Geometry: final body of the model. Coordinates: model frame, mm. A direction names the side the tool comes from. Round coordinates to 2 decimals unless told otherwise and drop trailing zeros. Write each loop counter-clockwise with the first axis right and the second up, starting at its lowest first coordinate (ties: lowest second). Pieces come first, ordered by that corner, then holes. Notation, with made-up numbers: (10.5, 1.25) - (30.5, 1.25) arc R22 cw to (30.5, 25.25) - close; hole circle Ø3 at (85.25, -38). An arc over 180 degrees is marked (long way). Use a Markdown table: item, result. Add a question column.
```python
from build123d import *

# Parameters (mm, degrees)
F0_W     = 3.175
F0_H     = 3.175
F0_H_2   = 6.35
F0_W_2   = 12.7
F1_DEPTH = 3.175
F2_W     = 19.05
F2_H     = 3.175
F3_DEPTH = 6.35
F4_W     = 6.35
F4_H     = 3.175
F5_DEPTH = 25.4


with BuildPart() as f1:
    # F0 (on Top) → F1 (new body)
    with BuildSketch(Plane.XY):
        with Locations((1.5875, 1.5875)):
            Rectangle(F0_W, F0_H)
        with Locations((1.5875, 6.35)):
            Rectangle(F0_W, F0_H_2)
        with Locations((1.5875, 11.1125)):
            Rectangle(F0_W, F0_H)
        with Locations((1.5875, 15.875)):
            Rectangle(F0_W, F0_H_2)
        with Locations((9.525, 11.1125)):
            Rectangle(F0_W_2, F0_H)
        with Locations((1.5875, 20.6375)):
            Rectangle(F0_W, F0_H)
        with Locations((17.4625, 6.35)):
            Rectangle(F0_W, F0_H_2)
        with Locations((17.4625, 11.1125)):
            Rectangle(F0_W, F0_H)
        with Locations((1.5875, 23.8125)):
            Rectangle(F0_W, F0_H)
        with Locations((9.525, 20.6375)):
            Rectangle(F0_W_2, F0_H)
        with Locations((17.4625, 15.875)):
            Rectangle(F0_W, F0_H_2)
        with Locations((17.4625, 1.5875)):
            Rectangle(F0_W, F0_H)
        with Locations((17.4625, 20.6375)):
            Rectangle(F0_W, F0_H)
        with Locations((17.4625, 23.8125)):
            Rectangle(F0_W, F0_H)
    extrude(amount=F1_DEPTH)

    # F2 (on face) → F3 (join)
    with BuildSketch(Plane(origin=(0, 0, 0), x_dir=(1, 0, 0), z_dir=(0, 0, -1))):
        with Locations((9.525, -26.9875)):
            Rectangle(F2_W, F2_H)
    extrude(amount=-F3_DEPTH)

    # F4 (on face) → F5 (cut)
    with BuildSketch(Plane(origin=(0, 28.575, 0), x_dir=(-1, 0, 0), z_dir=(0, 1, 0))):
        with Locations((-9.525, 4.7625)):
            Rectangle(F4_W, F4_H)
    extrude(amount=-F5_DEPTH, mode=Mode.SUBTRACT)


solid = f1.part
```
1) Section C-C, the plane y = 17. Return the cut outline in (x, z) (3 decimals).
2) Material intervals for L1, parallel to Y at x = 5.25, z = 2.75 (3 decimals); L2, parallel to X at y = 13, z = 2 (3 decimals); L3, parallel to Y at x = 1.75, z = 3.25 (3 decimals), sorted ascending. Write a range as from..to.
3) Set-up query: faces 3 (the flat face through (7, 10, 3.175)), 4 (the flat face through (15.875, 24, 2)), 5 (the flat face through (10, 27, 3.175)), 6 (the flat face through (9, 9.525, 2)), 7 (the flat face through (9, 25.4, 3)). Return all of +Z, -Z, +X, -X, +Y, -Y with unobstructed straight access to the full face (end or side cutting, diameter ignored); none if empty.
4) Section A-A, the plane z = 3.75. Return the cut outline in (x, y) (3 decimals), then the cut area to 3 significant figures.
5) Pin query (flat end, axial travel): P1, Ø1.6, axis at x = 12.5, z = 2, coming from the -Y side (3 decimals); P2, Ø1, axis at x = 8.5, y = 25.5, coming from the +Z side (3 decimals); P3, Ø1, axis at x = 7, z = 4, coming from the -Y side. Return the tip coordinate at first contact, or that it passes through.
6) Draft query along X for faces 1 (the flat face through (3.175, 16, 2)), 2 (the flat face through (3, 27, 6.35)). Return one class per face: released by +X, released by -X, zero draft, split by the parting line, or undercut.
7) Section D-D, the plane y = 26. Return the cut outline in (x, z) (3 decimals).
8) Section B-B, the plane x = 13.5. Return the cut outline in (y, z) (3 decimals).
Output values:
| question | item | result |
|---|---|---|
| 1 | outline | (0, 0) - (3.175, 0) - (3.175, 3.175) - (0, 3.175) - close; (15.875, 0) - (19.05, 0) - (19.05, 3.175) - (15.875, 3.175) - close |
| 2 | L1 | y = 9.525..12.7, 19.05..22.225, 25.4..28.575 |
| 2 | L2 | x = 0..3.175, 15.875..19.05 |
| 2 | L3 | y = 25.4..28.575 |
| 3 | face 3 | +Z, +X, -X, -Y |
| 3 | face 4 | +Z, -Z |
| 3 | face 5 | +Z, +Y, -Y |
| 3 | face 6 | +Z, -Z, -Y |
| 3 | face 7 | +Z |
| 4 | outline | (0, 25.4) - (6.35, 25.4) - (6.35, 28.575) - (0, 28.575) - close; (12.7, 25.4) - (19.05, 25.4) - (19.05, 28.575) - (12.7, 28.575) - close |
| 4 | area | 40.3 mm^2 |
| 5 | P1 | stops at y = 9.525 |
| 5 | P2 | stops at z = 3.175 |
| 5 | P3 | passes through |
| 6 | face 1 | undercut |
| 6 | face 2 | zero draft |
| 7 | outline | (0, 0) - (19.05, 0) - (19.05, 6.35) - (12.7, 6.35) - (12.7, 3.175) - (6.35, 3.175) - (6.35, 6.35) - (0, 6.35) - close |
| 8 | outline | (9.525, 0) - (12.7, 0) - (12.7, 3.175) - (9.525, 3.175) - close; (19.05, 0) - (22.225, 0) - (22.225, 3.175) - (19.05, 3.175) - close; (25.4, 0) - (28.575, 0) - (28.575, 6.35) - (25.4, 6.35) - close |
